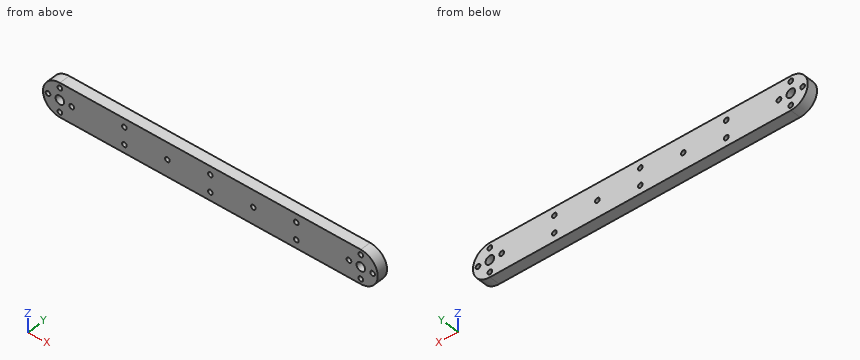
from build123d import *

# Parameters (mm, degrees)
SKETCH1_R           = 1.397
SKETCH1_R_2         = 2.54
BOSS_EXTRUDE1_DEPTH = 6.35


with BuildPart() as part:
    # Sketch1 → Boss-Extrude1 (new body)
    with BuildSketch(Plane(origin=(0, 0, 0), x_dir=(1, 0, 0), z_dir=(0, 1, 0))):
        with BuildLine():
            Line((0, 10), (177.8, 10))
            ThreePointArc((177.8, 10), (187.8, 0), (177.8, -10))
            Line((177.8, -10), (0, -10))
            ThreePointArc((0, -10), (-10, 0), (0, 10))
        make_face()
        with Locations(Location((-7, 0, 0), (0, 0, 270))):
            Circle(SKETCH1_R, mode=Mode.SUBTRACT)
        with Locations(Location((0, 0, 0), (0, 0, 270))):
            Circle(SKETCH1_R_2, mode=Mode.SUBTRACT)
        with Locations(Location((0, 7, 0), (0, 0, 270))):
            Circle(SKETCH1_R, mode=Mode.SUBTRACT)
        with Locations(Location((7, 0, 0), (0, 0, 270))):
            Circle(SKETCH1_R, mode=Mode.SUBTRACT)
        with Locations(Location((0, -7, 0), (0, 0, 270))):
            Circle(SKETCH1_R, mode=Mode.SUBTRACT)
        with Locations(Location((177.8, 7, 0), (0, 0, 90))):
            Circle(SKETCH1_R, mode=Mode.SUBTRACT)
        with Locations(Location((184.8, 0, 0), (0, 0, 90))):
            Circle(SKETCH1_R, mode=Mode.SUBTRACT)
        with Locations(Location((177.8, -7, 0), (0, 0, 90))):
            Circle(SKETCH1_R, mode=Mode.SUBTRACT)
        with Locations(Location((177.8, 0, 0), (0, 0, 90))):
            Circle(SKETCH1_R_2, mode=Mode.SUBTRACT)
        with Locations(Location((170.8, 0, 0), (0, 0, 90))):
            Circle(SKETCH1_R, mode=Mode.SUBTRACT)
        with Locations(Location((88.9, 5.08, 0), (0, 0, 270))):
            Circle(SKETCH1_R, mode=Mode.SUBTRACT)
        with Locations(Location((88.9, -5.08, 0), (0, 0, 90))):
            Circle(SKETCH1_R, mode=Mode.SUBTRACT)
        with Locations(Location((63.5, 0, 0), (0, 0, 270))):
            Circle(SKETCH1_R, mode=Mode.SUBTRACT)
        with Locations(Location((38.1, 5.08, 0), (0, 0, 90))):
            Circle(SKETCH1_R, mode=Mode.SUBTRACT)
        with Locations(Location((38.1, -5.08, 0), (0, 0, 270))):
            Circle(SKETCH1_R, mode=Mode.SUBTRACT)
        with Locations(Location((114.3, 0, 0), (0, 0, 90))):
            Circle(SKETCH1_R, mode=Mode.SUBTRACT)
        with Locations(Location((139.7, 5.08, 0), (0, 0, 270))):
            Circle(SKETCH1_R, mode=Mode.SUBTRACT)
        with Locations(Location((139.7, -5.08, 0), (0, 0, 90))):
            Circle(SKETCH1_R, mode=Mode.SUBTRACT)
    extrude(amount=BOSS_EXTRUDE1_DEPTH)


solid = part.part
Can you work these out from the model? Positions are in its coordinate system, mm. Coordinates: 2 decimals unless noted, no trailing zeros. Write each question's results on one line, items separated by ' | '. Start each with the question number.
Item 1: If we section it at A-A, the plane y = 2: Count the separate pieces of the cut face and the enclosed holes in it, and give its area (3 significant figures).
Item 2: I'm going to push flat-ended pins straight in: P1, Ø4.5, axis at x = 7, z = 0, coming from the -Y side; P2, Ø2.5, axis at x = 139.7, z = -5.08, coming from the -Y side; P3, Ø2, axis at y = 2, z = -1.5, coming from the +X side; P4, Ø1, axis at y = 0.5, z = 5, coming from the +X side. Where does each tip first touch, or does it pass through?
Item 3: Please list where these lines run through material, in increasing order: probe 1 along Z at (x, y) = (88.9, 4.25); probe 2 along Z at (x, y) = (177.8, 1.5); probe 3 along X at (y, z) = (3.75, -5).
Answer block:
1) separate pieces: 1 | enclosed holes: 18 | area: 3,730 mm²
2) P1: y = 0 | P2: through | P3: x = 187.79 | P4: x = 186.73
3) probe 1: -10 to -6.48, -3.68 to 3.68, 6.48 to 10 | probe 2: -10 to -8.4, -5.6 to -2.54, 2.54 to 5.6, 8.4 to 10 | probe 3: -8.66 to 36.71, 39.49 to 87.51, 90.29 to 138.31, 141.09 to 186.46
